For this review, take the finished solid that the model builds, in its own axes (mm). A direction names the side the tool comes from. Round coordinates to 2 decimals unless told otherwise and drop trailing zeros. Order: outer loops, then holes, each group sorted by start corner. A loop starts at its lowest first (then second) coordinate and runs counter-clockwise, first axis right, second up. Notation, with made-up numbers: M -9.5,45.25 L 8.5,45.25 A18 ccw 8.5,67.25 Z; hole C 68.25,66.25 d10. An arc over 180 degrees is marked long. Answer as a JSON object with one key per item and string values.
from build123d import *

# Parameters (mm, degrees)
EXTRUDE1_DEPTH             = 70
SKETCH2_R                  = 1.2
EXTRUDE2_DEPTH             = 5
SKETCH_R                   = 2.1
SKETCH_R_2                 = 1.2
EXTRUDE4_DEPTH             = 2.3
CHAMFER1_SIZE              = 0.2
LPATTERN1_COUNT            = 5
LPATTERN1_PITCH            = 15
CHAMFER1_OF_LPATTERN1_SIZE = 0.2


with BuildPart() as part:
    # Sketch1 → Extrude1 (new body)
    with BuildSketch(Plane.XY):
        with BuildLine():
            Line((-3.3, -2.5), (3.3, -2.5))
            Line((3.3, -2.5), (3.5, -2.3))
            Line((3.5, -2.3), (3.5, 0.206274607))
            ThreePointArc((3.5, 0.206274607), (3.091294745, 0.382570681), (2.840065792, 0.75))
            Line((2.840065792, 0.75), (2.340065792, 0.75))
            Line((2.340065792, 0.75), (2.340065792, 1.25))
            Line((2.340065792, 1.25), (2.840065792, 1.25))
            ThreePointArc((2.840065792, 1.25), (3.091294745, 1.617429319), (3.5, 1.793725393))
            Line((3.5, 1.793725393), (3.5, 2.3))
            Line((3.5, 2.3), (3.3, 2.5))
            Line((3.3, 2.5), (-3.3, 2.5))
            Line((-3.3, 2.5), (-3.5, 2.3))
            Line((-3.5, 2.3), (-3.5, 1.793725393))
            ThreePointArc((-3.5, 1.793725393), (-3.091294745, 1.617429319), (-2.840065792, 1.25))
            Line((-2.840065792, 1.25), (-2.340065792, 1.25))
            Line((-2.340065792, 1.25), (-2.340065792, 0.75))
            Line((-2.340065792, 0.75), (-2.840065792, 0.75))
            ThreePointArc((-2.840065792, 0.75), (-3.091294745, 0.382570681), (-3.5, 0.206274607))
            Line((-3.5, 0.206274607), (-3.5, -2.3))
            Line((-3.5, -2.3), (-3.3, -2.5))
        make_face()
    extrude(amount=EXTRUDE1_DEPTH)

    # Sketch2 → Extrude2 (cut)
    with BuildSketch(Plane(origin=(0, 2.5, 0), x_dir=(1, 0, 0), z_dir=(0, 1, 0))):
        with Locations((0, -5)):
            Circle(SKETCH2_R)
    extrude2 = extrude(amount=-EXTRUDE2_DEPTH, mode=Mode.SUBTRACT)

    # Sketch → Extrude4 (cut)
    with BuildSketch(Plane(origin=(0, 2.5, 0), x_dir=(1, 0, 0), z_dir=(0, 1, 0))):
        with Locations((0, -5)):
            Circle(SKETCH_R)
        with Locations((0, -5)):
            Circle(SKETCH_R_2, mode=Mode.SUBTRACT)
    extrude4 = extrude(amount=-EXTRUDE4_DEPTH, mode=Mode.SUBTRACT)

    # Chamfer1
    chamfer1_edges = [part.edges().sort_by_distance(p)[0] for p in [
        (-1.2, -2.5, 5),
        (-2.1, 2.5, 5),
    ]]
    chamfer(chamfer1_edges, length=CHAMFER1_SIZE)

    # LPattern1: Extrude2, Extrude4 ×5
    with Locations(*[(0, 0, i * LPATTERN1_PITCH) for i in range(1, LPATTERN1_COUNT)]):
        add(extrude2, mode=Mode.SUBTRACT)
        add(extrude4, mode=Mode.SUBTRACT)

    # Chamfer1 of LPattern1
    chamfer1_of_lpattern1_edges = [part.edges().sort_by_distance(p)[0] for p in [
        (-1.2, -2.5, 20),
        (-2.1, 2.5, 20),
        (-1.2, -2.5, 35),
        (-2.1, 2.5, 35),
        (-1.2, -2.5, 50),
        (-2.1, 2.5, 50),
        (-1.2, -2.5, 65),
        (-2.1, 2.5, 65),
    ]]
    chamfer(chamfer1_of_lpattern1_edges, length=CHAMFER1_OF_LPATTERN1_SIZE)


solid = part.part
1) Insertion check: P1, Ø2, axis at x = 0, z = 50, coming from the -Y side; P2, Ø1.3, axis at x = 0, z = 36, coming from the +Y side; P3, Ø3.5, axis at x = -0.5, z = 20, coming from the +Y side. Each pin has a flat end and moves straight along its axis. Give the tip position at first contact, or say it passes through.
Geometry check:
{"P1": "passes through", "P2": "stops at y = 0.2", "P3": "stops at y = 2.45"}
2) Add section D-D on x = 0. State how many separate pieces and enclosed holes the cut face has, and give its area (3 significant figures).
Geometry check:
{"separate pieces": "6", "enclosed holes": "0", "area": "269 mm²"}
3) Add section B-B on y = -0.85. State the section outline as (x, z) points.
Geometry check:
{"outline": "M -3.5,0 L 3.5,0 L 3.5,70 L -3.5,70 Z; hole C 0,5 d2.4; hole C 0,20 d2.4; hole C 0,35 d2.4; hole C 0,50 d2.4; hole C 0,65 d2.4"}
4) Machinability: for faces 3 (the cylindrical face through (-0.16, -1.03, 48.81)), 4 (the flat face through (1, 0.2, 36)), which of the approach directions +Z, -Z, +X, -X, +Y, -Y give a long, thin tool a straight path to every point of the face, cutting with its end or side? Answer none if there is none.
Geometry check:
{"face 3": "+Y, -Y", "face 4": "+Y"}
5) Mouldability with a two-part tool opening along Z and no side actions: class faces 1 (the flat face through (3, 2.5, 35)), 2 (the flat face through (1, 0.2, 51)) as +Z half, -Z half, draft (parallel to the pull), parting line (faces both ways), or undercut.
Geometry check:
{"face 1": "draft", "face 2": "undercut"}
6) Add section A-A on z = 17. State the section outline as (x, y) points, and give its area (3 significant figures).
Geometry check:
{"outline": "M -3.5,-2.3 L -3.3,-2.5 L 3.3,-2.5 L 3.5,-2.3 L 3.5,0.21 A0.8 cw 2.84,0.75 L 2.34,0.75 L 2.34,1.25 L 2.84,1.25 A0.8 cw 3.5,1.79 L 3.5,2.3 L 3.3,2.5 L -3.3,2.5 L -3.5,2.3 L -3.5,1.79 A0.8 cw -2.84,1.25 L -2.34,1.25 L -2.34,0.75 L -2.84,0.75 A0.8 cw -3.5,0.21 Z", "area": "32.8 mm²"}
7) For L1, parallel to Z at x = 0, y = -1.55; L2, parallel to Z at x = 0, y = 1.6; L3, parallel to X at y = -1.25, z = 35, list the stretches that pass through material, from the lowest coordinate up.
Geometry check:
{"L1": "z = 0 to 3.8, 6.2 to 18.8, 21.2 to 33.8, 36.2 to 48.8, 51.2 to 63.8, 66.2 to 70", "L2": "z = 0 to 2.9, 7.1 to 17.9, 22.1 to 32.9, 37.1 to 47.9, 52.1 to 62.9, 67.1 to 70", "L3": "x = -3.5 to -1.2, 1.2 to 3.5"}
